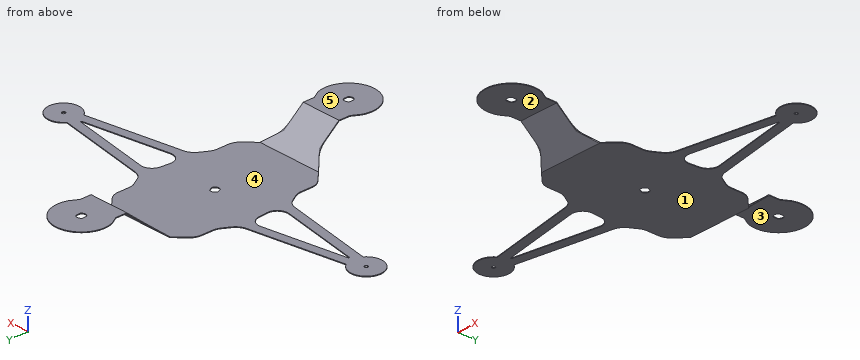
```python
from build123d import *

# Parameters (mm, degrees)
SALIENTE_EXTRUIR1_DEPTH     = 271
CORTAR_EXTRUIR9_DEPTH       = 372.904084134
CORTAR_EXTRUIR9_DEPTH_BACK  = 372.904084134
CROQUIS4_R                  = 2.5
CORTAR_EXTRUIR10_DEPTH      = 372.904084134
CORTAR_EXTRUIR10_DEPTH_BACK = 372.904084134
CROQUIS2_W                  = 581.580028242
CROQUIS2_H                  = 554.061756016
REDONDEO1_R                 = 20
REDONDEO2_R                 = 15
REDONDEO3_R                 = 1


with BuildPart() as part:
    # Croquis1 → Saliente-Extruir1 (new, symmetric)
    with BuildSketch(Plane(origin=(0, 0, 0), x_dir=(0, 0, -1), z_dir=(1, 0, 0))):
        Polygon((-18.5, -110), (-18.5, 110), (-58.031437996, 157.111733252), (-58.031437996, 248), (-57.031437996, 248), (-57.031437996, 157.475703486), (-17.5, 110.363970234), (-17.5, -110.363970234), (-57.031437996, -157.475703486), (-57.031437996, -248), (-58.031437996, -248), (-58.031437996, -157.111733252), align=None)
    extrude(amount=SALIENTE_EXTRUIR1_DEPTH, both=True)

    # Croquis4 → Cortar-Extruir9 (cut, two sides: drawn at the far end of the back side and taken through both)
    with BuildSketch(Plane.XY.offset(-CORTAR_EXTRUIR9_DEPTH_BACK)):
        with Locations(Location((-242, 0, 0), (0, 0, 90))):
            Circle(CROQUIS4_R)
        with Locations(Location((242, 0, 0), (0, 0, 90))):
            Circle(CROQUIS4_R)
        with BuildLine():
            Line((-5, 201.31662479), (-5, 194.68337521))
            ThreePointArc((-5, 194.68337521), (0, 192), (5, 194.68337521))
            Line((5, 194.68337521), (5, 201.31662479))
            ThreePointArc((5, 201.31662479), (0, 204), (-5, 201.31662479))
        make_face()
        with BuildLine():
            Line((5, -201.31662479), (5, -194.68337521))
            ThreePointArc((5, -194.68337521), (0, -192), (-5, -194.68337521))
            Line((-5, -194.68337521), (-5, -201.31662479))
            ThreePointArc((-5, -201.31662479), (0, -204), (5, -201.31662479))
        make_face()
        with BuildLine():
            Line((-5.933205139, 0.892791565), (-3.129872731, -5.118974183))
            ThreePointArc((-3.129872731, -5.118974183), (2.53570957, -5.437846722), (5.933205139, -0.892791565))
            Line((5.933205139, -0.892791565), (3.129872731, 5.118974183))
            ThreePointArc((3.129872731, 5.118974183), (-2.53570957, 5.437846722), (-5.933205139, 0.892791565))
        make_face()
    extrude(amount=CORTAR_EXTRUIR9_DEPTH + CORTAR_EXTRUIR9_DEPTH_BACK, mode=Mode.SUBTRACT)

    # Croquis2 → Cortar-Extruir10 (cut, two sides: drawn at the far end of the back side and taken through both)
    # profile 1 of 3: a face of its own
    with BuildSketch(Plane.XY.offset(-CORTAR_EXTRUIR10_DEPTH_BACK)):
        Rectangle(CROQUIS2_W, CROQUIS2_H)
        with BuildLine():
            Line((80, 37.378360334), (223.291713066, 12.5))
            ThreePointArc((223.291713066, 12.5), (264.5, 0), (223.291713066, -12.5))
            Line((223.291713066, -12.5), (80, -37.378360334))
            Line((80, -37.378360334), (66.939390249, -60))
            Line((66.939390249, -60), (66.939390249, -89.839367484))
            Line((66.939390249, -89.839367484), (28.5, -128.278757733))
            Line((28.5, -128.278757733), (28.5, -173.278757733))
            Line((28.5, -173.278757733), (35, -184.537087982))
            ThreePointArc((35, -184.537087982), (0, -235.5), (-35, -184.537087982))
            Line((-35, -184.537087982), (-28.5, -173.278757733))
            Line((-28.5, -173.278757733), (-28.5, -128.278757733))
            Line((-28.5, -128.278757733), (-66.939390249, -89.839367484))
            Line((-66.939390249, -89.839367484), (-66.939390249, -60))
            Line((-66.939390249, -60), (-80, -37.378360334))
            Line((-80, -37.378360334), (-223.291713066, -12.5))
            ThreePointArc((-223.291713066, -12.5), (-264.5, 0), (-223.291713066, 12.5))
            Line((-223.291713066, 12.5), (-80, 37.378360334))
            Line((-80, 37.378360334), (-66.939390249, 60))
            Line((-66.939390249, 60), (-66.939390249, 89.839367484))
            Line((-66.939390249, 89.839367484), (-28.5, 128.278757733))
            Line((-28.5, 128.278757733), (-28.5, 173.278757733))
            Line((-28.5, 173.278757733), (-35, 184.537087982))
            ThreePointArc((-35, 184.537087982), (0, 235.5), (35, 184.537087982))
            Line((35, 184.537087982), (28.5, 173.278757733))
            Line((28.5, 173.278757733), (28.5, 128.278757733))
            Line((28.5, 128.278757733), (66.939390249, 89.839367484))
            Line((66.939390249, 89.839367484), (66.939390249, 60))
            Line((66.939390249, 60), (80, 37.378360334))
        make_face(mode=Mode.SUBTRACT)
    # profile 2 of 3: a face of its own
    with BuildSketch(Plane.XY.offset(-CORTAR_EXTRUIR10_DEPTH_BACK)):
        Polygon((-75.703100415, -24.92990815), (-80, -24.183878851), (-219.291713066, 0), (-80, 24.183878851), align=None)
    # profile 3 of 3: a face of its own
    with BuildSketch(Plane.XY.offset(-CORTAR_EXTRUIR10_DEPTH_BACK)):
        Polygon((80, 24.183878851), (75.703100415, -24.92990815), (80, -24.183878851), (219.291713066, 0), align=None)
    extrude(amount=CORTAR_EXTRUIR10_DEPTH + CORTAR_EXTRUIR10_DEPTH_BACK, mode=Mode.SUBTRACT)

    # Redondeo1
    # the kernel refuses this fillet: 20 mm, written as the material it adds along each edge
    with BuildSketch(Plane(origin=(-28.5, 128.278757733, 54.548376991), x_dir=(-0.7071067811865487, -0.7071067811865461, 0), z_dir=(0, 0, -1))) as redondeo1_piece_1_section:
        with BuildLine():
            CenterArc((REDONDEO1_R * 0.414213562373, REDONDEO1_R), REDONDEO1_R, 225, 45)
            Line((-REDONDEO1_R * 0.292893218813, REDONDEO1_R * 0.292893218813), (0, 0))
            Line((0, 0), (REDONDEO1_R * 0.414213562373, 0))
        make_face()
    redondeo1_piece_1 = extrude(amount=42.726763527, mode=Mode.PRIVATE)
    redondeo1_piece_1 = split(redondeo1_piece_1, bisect_by=Plane(origin=(-29.703304355, 128.455788912, 33.986245669), z_dir=(0, 0.6427876096865383, -0.7660444431189789)), keep=Keep.TOP, mode=Mode.PRIVATE)
    redondeo1_piece_1 = split(redondeo1_piece_1, bisect_by=Plane(origin=(-29.703304355, 129.098576521, 33.220201226), z_dir=(0, -0.6427876096865383, 0.766044443118979)), keep=Keep.TOP, mode=Mode.PRIVATE)
    add(redondeo1_piece_1)
    with BuildSketch(Plane(origin=(80, 37.378360334, 18.5), x_dir=(0.9852603921679417, -0.17106127447518257, 0), z_dir=(0, 0, -1)), Plane(origin=(80, -37.378360334, 18.5), x_dir=(-0.5000000000000011, -0.8660254037844379, 0), z_dir=(0, 0, -1)), Plane(origin=(-80, -37.378360334, 18.5), x_dir=(-0.9852603921679428, 0.17106127447517586, 0), z_dir=(0, 0, -1)), Plane(origin=(-80, 37.378360334, 18.5), x_dir=(0.5000000000000069, 0.8660254037844347, 0), z_dir=(0, 0, -1))) as redondeo1_piece_2:
        with BuildLine():
            CenterArc((REDONDEO1_R * 0.467907265941, -REDONDEO1_R), REDONDEO1_R, 90, 50.15047048)
            Line((-REDONDEO1_R * 0.299822625782, -REDONDEO1_R * 0.359226394617), (0, 0))
            Line((0, 0), (REDONDEO1_R * 0.467907265941, 0))
        make_face()
    extrude(amount=1)
    with BuildSketch(Plane(origin=(66.939390249, -60, 18.5), x_dir=(0, -1, 0), z_dir=(0, 0, -1)), Plane(origin=(-66.939390249, -60, 18.5), x_dir=(-0.5000000000000052, 0.8660254037844356, 0), z_dir=(0, 0, -1)), Plane(origin=(-66.939390249, 60, 18.5), x_dir=(0, 1, 0), z_dir=(0, 0, -1)), Plane(origin=(66.939390249, 60, 18.5), x_dir=(0.5000000000000032, -0.8660254037844367, 0), z_dir=(0, 0, -1))) as redondeo1_piece_3:
        with BuildLine():
            CenterArc((REDONDEO1_R * 0.267949192431, -REDONDEO1_R), REDONDEO1_R, 90, 30)
            Line((-REDONDEO1_R * 0.232050807569, -REDONDEO1_R * 0.133974596216), (0, 0))
            Line((0, 0), (REDONDEO1_R * 0.267949192431, 0))
        make_face()
    extrude(amount=1)
    with BuildSketch(Plane(origin=(28.5, 128.278757733, 54.548376991), x_dir=(0.7071067811865498, -0.7071067811865451, 0), z_dir=(0, 0, -1))) as redondeo1_piece_4_section:
        with BuildLine():
            CenterArc((REDONDEO1_R * 0.414213562373, -REDONDEO1_R), REDONDEO1_R, 90, 45)
            Line((-REDONDEO1_R * 0.292893218813, -REDONDEO1_R * 0.292893218813), (0, 0))
            Line((0, 0), (REDONDEO1_R * 0.414213562373, 0))
        make_face()
    redondeo1_piece_4 = extrude(amount=42.726763527, mode=Mode.PRIVATE)
    redondeo1_piece_4 = split(redondeo1_piece_4, bisect_by=Plane(origin=(29.703304355, 128.455788912, 33.986245669), z_dir=(0, 0.6427876096865383, -0.7660444431189789)), keep=Keep.TOP, mode=Mode.PRIVATE)
    redondeo1_piece_4 = split(redondeo1_piece_4, bisect_by=Plane(origin=(29.703304355, 129.098576521, 33.220201226), z_dir=(0, -0.6427876096865383, 0.766044443118979)), keep=Keep.TOP, mode=Mode.PRIVATE)
    add(redondeo1_piece_4)
    with BuildSketch(Plane(origin=(28.5, -128.278757733, 54.548376991), x_dir=(0.7071067811865518, 0.7071067811865431, 0), z_dir=(0, 0, -1))) as redondeo1_piece_5_section:
        with BuildLine():
            CenterArc((REDONDEO1_R * 0.414213562373, REDONDEO1_R), REDONDEO1_R, 225, 45)
            Line((-REDONDEO1_R * 0.292893218813, REDONDEO1_R * 0.292893218813), (0, 0))
            Line((0, 0), (REDONDEO1_R * 0.414213562373, 0))
        make_face()
    redondeo1_piece_5 = extrude(amount=42.726763527, mode=Mode.PRIVATE)
    redondeo1_piece_5 = split(redondeo1_piece_5, bisect_by=Plane(origin=(29.703304355, -128.455788912, 33.986245669), z_dir=(0, -0.6427876096865381, -0.766044443118979)), keep=Keep.TOP, mode=Mode.PRIVATE)
    redondeo1_piece_5 = split(redondeo1_piece_5, bisect_by=Plane(origin=(29.703304355, -129.098576521, 33.220201226), z_dir=(0, 0.6427876096865377, 0.7660444431189795)), keep=Keep.TOP, mode=Mode.PRIVATE)
    add(redondeo1_piece_5)
    with BuildSketch(Plane(origin=(-28.5, -128.278757733, 54.548376991), x_dir=(-0.7071067811865503, 0.7071067811865448, 0), z_dir=(0, 0, -1))) as redondeo1_piece_6_section:
        with BuildLine():
            CenterArc((REDONDEO1_R * 0.414213562373, -REDONDEO1_R), REDONDEO1_R, 90, 45)
            Line((-REDONDEO1_R * 0.292893218813, -REDONDEO1_R * 0.292893218813), (0, 0))
            Line((0, 0), (REDONDEO1_R * 0.414213562373, 0))
        make_face()
    redondeo1_piece_6 = extrude(amount=42.726763527, mode=Mode.PRIVATE)
    redondeo1_piece_6 = split(redondeo1_piece_6, bisect_by=Plane(origin=(-29.703304355, -128.455788912, 33.986245669), z_dir=(0, -0.6427876096865381, -0.766044443118979)), keep=Keep.TOP, mode=Mode.PRIVATE)
    redondeo1_piece_6 = split(redondeo1_piece_6, bisect_by=Plane(origin=(-29.703304355, -129.098576521, 33.220201226), z_dir=(0, 0.6427876096865377, 0.7660444431189795)), keep=Keep.TOP, mode=Mode.PRIVATE)
    add(redondeo1_piece_6)
    # the kernel refuses this fillet: 20 mm, written as the material it takes off along each edge
    with BuildSketch(Plane(origin=(-66.939390249, -89.839367484, 39.210678119), x_dir=(0, 1, 0), z_dir=(0, 0, -1)), Plane(origin=(-66.939390249, 89.839367484, 39.210678119), x_dir=(0.7071067811865483, 0.7071067811865467, 0), z_dir=(0, 0, -1)), Plane(origin=(66.939390249, 89.839367484, 39.210678119), x_dir=(0, -1, 0), z_dir=(0, 0, -1)), Plane(origin=(66.939390249, -89.839367484, 39.210678119), x_dir=(-0.7071067811865501, -0.707106781186545, 0), z_dir=(0, 0, -1))) as redondeo1_2_piece_1:
        with BuildLine():
            CenterArc((REDONDEO1_R * 0.414213562373, REDONDEO1_R), REDONDEO1_R, 225, 45)
            Line((-REDONDEO1_R * 0.292893218813, REDONDEO1_R * 0.292893218813), (0, 0))
            Line((0, 0), (REDONDEO1_R * 0.414213562373, 0))
        make_face()
    extrude(amount=42.421356237, mode=Mode.SUBTRACT)

    # Redondeo2
    redondeo2_edges = [part.edges().sort_by_distance(p)[0] for p in [
        (80, 24.183878851, 18),
        (75.703100415, -24.92990815, 18),
        (-75.703100415, -24.92990815, 18),
        (-80, 24.183878851, 18),
    ]]
    fillet(redondeo2_edges, radius=REDONDEO2_R)

    # Redondeo3
    redondeo3_edges = [part.edges().sort_by_distance(p)[0] for p in [
        (219.291713066, 0, 18),
        (-219.291713066, 0, 18),
    ]]
    fillet(redondeo3_edges, radius=REDONDEO3_R)


solid = part.part
```
CAD build for the part. Positions are in the model's coordinates, mm. Face numbers are marked on the shaded views. A direction names the side the tool comes from. Round coordinates to 2 decimals unless told otherwise and drop trailing zeros. Write each loop counter-clockwise with the first axis right and the second up, starting at its lowest first coordinate (ties: lowest second). Pieces come first, ordered by that corner, then holes. Notation, with made-up numbers: (32, 35.25) -> (38, 35.25) arc R15 cw to (38, 45.25) -> close; hole circle Ø7 at (-39.75, 82). An arc over 180 degrees is marked (long way). Answer in a Markdown table with one row per item. Add a question column.
Item 1: Drop flat-ended pins along their axis: pin 1 Ø9.5 at (y, z) = (163.5, 51.5) entering from -X; pin 2 Ø5.5 at (y, z) = (-147, 47.5) entering from +X; pin 3 Ø3 at (x, y) = (12.5, -135) entering from -Z; pin 4 Ø0.8 at (y, z) = (-197, 57.5) entering from +X. Give the stop position or say it passes through.
Item 2: Mould opens along Y. For the marked faces 4 and 5 say: pulls with the +Y half, pulls with the -Y half, needs draft (parallel to the pull), parting line crosses it, or undercut.
Item 3: Drill centre lines: line 1 (Y direction, x = -242, z = 18); line 2 (Z direction, x = 26.5, y = -8); line 3 (Y direction, x = 12.5, z = 48). Where is each one in solid material? Low to high. Write a range as from..to.
Item 4: Which spindle directions (+Z, -Z, +X, -X, +Y, -Y) get a long thin tool onto all of the face, cutting with end or side? Do the marked faces 1, 2 and 3. Say none if no direction does.
Item 5: Saw through at A-A, the plane x = -111. Write the cut outline in (y, z), then the cut area to 3 significant figures.
Findings below:
| question | item | result |
|---|---|---|
| 1 | pin 1 | passes through |
| 1 | pin 2 | stops at x = 28.5 |
| 1 | pin 3 | stops at z = 36.91 |
| 1 | pin 4 | stops at x = 37.5 |
| 2 | face 4 | undercut |
| 2 | face 5 | needs draft |
| 3 | line 1 | y = -22.5..-2.5, 2.5..22.5 |
| 3 | line 2 | z = 17.5..18.5 |
| 3 | line 3 | y = -146.71..-145.16, 145.16..146.71 |
| 4 | face 1 | -Z, +X, -X, +Y, -Y |
| 4 | face 2 | -Z, +X, -X, -Y |
| 4 | face 3 | -Z, +X, -X, +Y |
| 5 | outline | (-32, 17.5) -> (-18.8, 17.5) -> (-18.8, 18.5) -> (-32, 18.5) -> close; (18.8, 17.5) -> (32, 17.5) -> (32, 18.5) -> (18.8, 18.5) -> close |
| 5 | area | 26.4 mm^2 |
